from build123d import *

# Parameters (mm, degrees)
SKETCH_3_R      = 2.2
SKETCH_3_R_2    = 1.5
EXTRUDE_1_DEPTH = 2


with BuildPart() as part:
    # 草图3 → 凸台-拉伸1 (new body)
    with BuildSketch(Plane.XY):
        with BuildLine():
            Line((-47, 31.317051182), (-47, -93.890216685))
            Line((-47, -93.890216685), (-45, -97.990216685))
            ThreePointArc((-45, -97.990216685), (-44.707106781, -98.697323466), (-44, -98.990216685))
            Line((-44, -98.990216685), (-25.9, -98.990216685))
            Line((-25.9, -98.990216685), (-25.9, -97.990216685))
            Line((-25.9, -97.990216685), (-25.9, -93.890216685))
            Line((-25.9, -93.890216685), (-31.748789112, -78.174983751))
            ThreePointArc((-31.748789112, -78.174983751), (-31.936696359, -77.488601938), (-32, -76.779784772))
            Line((-32, -76.779784772), (-32, -5.5))
            ThreePointArc((-32, -5.5), (-30.828427125, -2.671572875), (-28, -1.5))
            Line((-28, -1.5), (28, -1.5))
            ThreePointArc((28, -1.5), (30.828427125, -2.671572875), (32, -5.5))
            Line((32, -5.5), (32, -76.779784772))
            ThreePointArc((32, -76.779784772), (31.936696359, -77.488601938), (31.748789112, -78.174983751))
            Line((31.748789112, -78.174983751), (25.9, -93.890216685))
            Line((25.9, -93.890216685), (25.9, -97.990216685))
            Line((25.9, -97.990216685), (25.9, -98.990216685))
            Line((25.9, -98.990216685), (45, -98.990216685))
            Line((45, -98.990216685), (47, -93.890216685))
            Line((47, -93.890216685), (47, 31.741152315))
            Line((47, 31.741152315), (45.230037269, 31.741152315))
            ThreePointArc((45.230037269, 31.741152315), (36.686440181, 34.468680322), (28.716551195, 30.356098435))
            ThreePointArc((28.716551195, 30.356098435), (27.478316584, 29.033500084), (26.179230338, 27.770619934))
            ThreePointArc((26.179230338, 27.770619934), (16.152230905, 17.515551518), (1.809761925, 17.542559084))
            ThreePointArc((1.809761925, 17.542559084), (0, 17.5), (-1.809761925, 17.542559084))
            ThreePointArc((-1.809761925, 17.542559084), (-15.928828372, 17.542283516), (-25.912710857, 27.525776288))
            ThreePointArc((-25.912710857, 27.525776288), (-27.223611076, 28.776388924), (-28.474223712, 30.087289143))
            ThreePointArc((-28.474223712, 30.087289143), (-36.482419799, 34.124770496), (-45, 31.317051182))
            Line((-45, 31.317051182), (-47, 31.317051182))
        make_face()
        with Locations((0, 13.5)):
            Circle(SKETCH_3_R, mode=Mode.SUBTRACT)
        with Locations((-30.052038202, 25.947961669)):
            Circle(SKETCH_3_R, mode=Mode.SUBTRACT)
        with Locations((30.199957913, 26.082571452)):
            Circle(SKETCH_3_R, mode=Mode.SUBTRACT)
        with Locations((42.5, -14.940216685)):
            Circle(SKETCH_3_R_2, mode=Mode.SUBTRACT)
        with Locations(Location((-42.5, -14.940216685, 0), (0, 0, 180))):
            Circle(SKETCH_3_R_2, mode=Mode.SUBTRACT)
        with Locations((42.5, -84.940216685)):
            Circle(SKETCH_3_R_2, mode=Mode.SUBTRACT)
        with Locations((-42.5, -84.940216685)):
            Circle(SKETCH_3_R_2, mode=Mode.SUBTRACT)
        with BuildLine():
            Line((-37.1, -96.090216685), (-29.9, -96.090216685))
            Line((-29.9, -96.090216685), (-29.9, -93.890216685))
            Line((-29.9, -93.890216685), (-37.1, -93.890216685))
            ThreePointArc((-37.1, -93.890216685), (-37.555634919, -94.990216685), (-37.1, -96.090216685))
        make_face(mode=Mode.SUBTRACT)
        with BuildLine():
            Line((-41.45513954, -19.890216685), (-41.45513954, -25.190216685))
            Line((-41.45513954, -25.190216685), (-43.65513954, -25.190216685))
            Line((-43.65513954, -25.190216685), (-43.65513954, -19.890216685))
            ThreePointArc((-43.65513954, -19.890216685), (-42.55513954, -19.434581767), (-41.45513954, -19.890216685))
        make_face(mode=Mode.SUBTRACT)
        with BuildLine():
            Line((37.1, -93.890216685), (29.9, -93.890216685))
            Line((29.9, -93.890216685), (29.9, -96.090216685))
            Line((29.9, -96.090216685), (37.1, -96.090216685))
            ThreePointArc((37.1, -96.090216685), (37.555634919, -94.990216685), (37.1, -93.890216685))
        make_face(mode=Mode.SUBTRACT)
        with BuildLine():
            Line((43.54486046, -25.190216685), (43.54486046, -19.890216685))
            ThreePointArc((43.54486046, -19.890216685), (42.44486046, -19.434581767), (41.34486046, -19.890216685))
            Line((41.34486046, -19.890216685), (41.34486046, -25.190216685))
            Line((41.34486046, -25.190216685), (43.54486046, -25.190216685))
        make_face(mode=Mode.SUBTRACT)
        with BuildLine():
            Line((41.34486046, -9.990216685), (41.34486046, -4.690216685))
            Line((41.34486046, -4.690216685), (43.54486046, -4.690216685))
            Line((43.54486046, -4.690216685), (43.54486046, -9.990216685))
            ThreePointArc((43.54486046, -9.990216685), (42.44486046, -10.445851604), (41.34486046, -9.990216685))
        make_face(mode=Mode.SUBTRACT)
        with BuildLine():
            Line((43.6, -95.190216685), (43.6, -89.890216685))
            ThreePointArc((43.6, -89.890216685), (42.5, -89.434581767), (41.4, -89.890216685))
            Line((41.4, -89.890216685), (41.4, -95.190216685))
            Line((41.4, -95.190216685), (43.6, -95.190216685))
        make_face(mode=Mode.SUBTRACT)
        with BuildLine():
            Line((41.4, -74.890216685), (41.4, -80.090216685))
            ThreePointArc((41.4, -80.090216685), (42.5, -80.545851604), (43.6, -80.090216685))
            Line((43.6, -80.090216685), (43.6, -74.890216685))
            Line((43.6, -74.890216685), (41.4, -74.890216685))
        make_face(mode=Mode.SUBTRACT)
        with BuildLine():
            Line((-41.4, -95.190216685), (-41.4, -89.890216685))
            ThreePointArc((-41.4, -89.890216685), (-42.5, -89.434581767), (-43.6, -89.890216685))
            Line((-43.6, -89.890216685), (-43.6, -95.190216685))
            Line((-43.6, -95.190216685), (-41.4, -95.190216685))
        make_face(mode=Mode.SUBTRACT)
        with BuildLine():
            Line((-43.6, -74.890216685), (-43.6, -80.090216685))
            ThreePointArc((-43.6, -80.090216685), (-42.5, -80.545851604), (-41.4, -80.090216685))
            Line((-41.4, -80.090216685), (-41.4, -74.890216685))
            Line((-41.4, -74.890216685), (-43.6, -74.890216685))
        make_face(mode=Mode.SUBTRACT)
        with BuildLine():
            Line((-43.65513954, -4.690216685), (-43.65513954, -9.990216685))
            ThreePointArc((-43.65513954, -9.990216685), (-42.55513954, -10.445851604), (-41.45513954, -9.990216685))
            Line((-41.45513954, -9.990216685), (-41.45513954, -4.690216685))
            Line((-41.45513954, -4.690216685), (-43.65513954, -4.690216685))
        make_face(mode=Mode.SUBTRACT)
    extrude(amount=EXTRUDE_1_DEPTH)


solid = part.part
Can you work these out from the model? Positions are in its coordinate system, mm. A direction names the side the tool comes from. Coordinates: 2 decimals unless noted, no trailing zeros. Order: outer loops, then holes, each group sorted by start corner. A loop starts at its lowest first (then second) coordinate and runs counter-clockwise, first axis right, second up. Notation, with made-up numbers: (64, 53.25) -> (72, 53.25) arc R25 cw to (72, 76.25) -> close; hole circle Ø10 at (8, 48.5). An arc over 180 degrees is marked (long way). Use one line per item in the form item = value.
Q1. Imagine slicing it at D-D, the plane z = 0.5. Give the number of separate pieces and of enclosed holes in the cut face, then the cut area to 3 significant figures.
From the geometry:
separate_pieces = 1
enclosed_holes = 17
area = 5,340 mm²
Q2. I need wall thicknesses on L1, parallel to X at y = -75.5, z = 0.5; L2, parallel to X at y = -42.5, z = 0.6; L3, parallel to X at y = -77.5, z = 1.7. Which ranges of each line are inside material? Lowest first, please.
From the geometry:
L1 = -47 to -43.6, -41.4 to -32, 32 to 41.4, 43.6 to 47
L2 = -47 to -32, 32 to 47
L3 = -47 to -43.6, -41.4 to -31.93, 31.93 to 41.4, 43.6 to 47
Q3. Imagine slicing it at C-C, the plane y = -23. List the corners of the cut face in (x, z) for me, then the cut area to 3 significant figures.
From the geometry:
outline = (-47, 0) -> (-43.66, 0) -> (-43.66, 2) -> (-47, 2) -> close; (-41.46, 0) -> (-32, 0) -> (-32, 2) -> (-41.46, 2) -> close; (32, 0) -> (41.34, 0) -> (41.34, 2) -> (32, 2) -> close; (43.54, 0) -> (47, 0) -> (47, 2) -> (43.54, 2) -> close
area = 51.2 mm²
Q4. Which directions (+Z, -Z, +X, -X, +Y, -Y) give clear straight access to the entire face, cutting with the end or side of a thin tool? Please do faces 1 (the face through (-30.859, -2.703, 0.986)), 2 (the face through (27.496, 29.052, 0.986)), 3 (the face through (3, 3, 2)).
From the geometry:
face_1 = +Z, -Z
face_2 = +Z, -Z, +Y
face_3 = +Z, +X, -X, +Y, -Y
Q5. We'd pull the mould along Y, two halves only. Please class faces 4 (the face through (41, -15, 1)), 5 (the face through (3, 3, 0)), 6 (the face through (-27.21, 28.76, 0.99)): released by +Y, released by -Y, zero draft, split by the parting line, or undercut.
From the geometry:
face_4 = undercut
face_5 = zero draft
face_6 = released by +Y
Q6. Imagine slicing it at A-A, the plane y = -61.5. List the corners of the cut face in (x, z) for me, then the cut area to 3 significant figures.
From the geometry:
outline = (-47, 0) -> (-32, 0) -> (-32, 2) -> (-47, 2) -> close; (32, 0) -> (47, 0) -> (47, 2) -> (32, 2) -> close
area = 60.0 mm²
Q7. Imagine slicing it at B-B, the plane x = 0. List the corners of the cut face in (y, z) for me, then the cut area to 3 significant figures.
From the geometry:
outline = (-1.5, 0) -> (11.3, 0) -> (11.3, 2) -> (-1.5, 2) -> close; (15.7, 0) -> (17.5, 0) -> (17.5, 2) -> (15.7, 2) -> close
area = 29.2 mm²
Q8. Will these pins go through, and if not, where does the flat tip stop? P1, Ø1, axis at x = 35, z = 0.5, coming from the +Y side; P2, Ø2.5, axis at x = -42.5, y = -14.94, coming from the -Z side; P3, Ø1, axis at y = -94.5, z = 1.5, coming from the +X side; P4, Ø0.6, axis at y = -96.5, z = 1.5, coming from the -X side.
From the geometry:
P1 = 34.31
P2 = through
P3 = 46.96
P4 = -45.87
